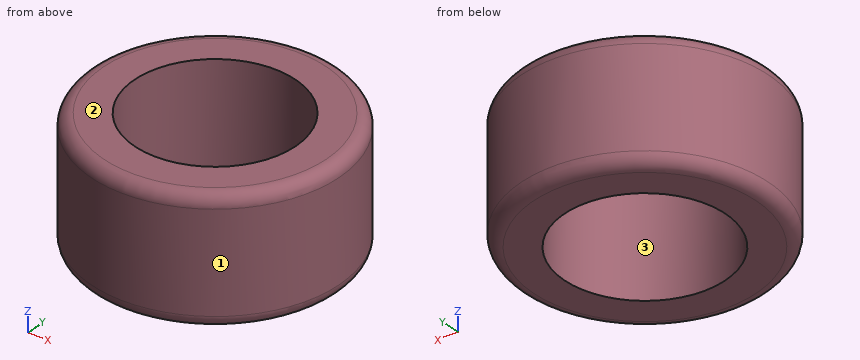
```python
from build123d import *

# Parameters (mm, degrees)
F0_R     = 10
F0_R_2   = 6.5
F1_DEPTH = 10
F2_R     = 1
F3_R     = 1


with BuildPart() as f1:
    # F0 (on Top) → F1 (new body)
    with BuildSketch(Plane.XY):
        Circle(F0_R)
        Circle(F0_R_2, mode=Mode.SUBTRACT)
    extrude(amount=F1_DEPTH)

    # F2
    f2_edges = [f1.edges().sort_by_distance(p)[0] for p in [
        (-10, 0, 10),
    ]]
    fillet(f2_edges, radius=F2_R)

    # F3
    f3_edges = [f1.edges().sort_by_distance(p)[0] for p in [
        (-10, 0, 0),
    ]]
    fillet(f3_edges, radius=F3_R)


solid = f1.part
```
Can you work these out from the model? Positions are in its coordinate system, mm. Face numbers are marked on the shaded views. Round coordinates to 2 decimals unless told otherwise and drop trailing zeros. Loops run counter-clockwise (first coordinate to the right, second up) from the corner with the lowest first, then second, coordinate; pieces in that order, holes last. Notation, with made-up numbers: M 11,13 L 46,13 A25 ccw 46,39 Z; hole C 19.25,-13.75 d3. An arc over 180 degrees is marked long. Write item = value, one per line. Start each with the question number.
(1) If we mould it in two halves opening along X, with no side actions, what happens to the marked faces 1, 2 and 3? For each: released by +X, released by -X, zero draft, split by the parting line, or undercut.
(2) I'm going to push flat-ended pins straight in: P1, Ø6, axis at y = -7.5, z = 4.5, coming from the -X side; P2, Ø1, axis at x = -3.5, z = 4.5, coming from the +Y side; P3, Ø2, axis at y = 1.5, z = 3.5, coming from the -X side. Where does each tip first touch, or does it pass through?
(3) Suppose I cut it at A-A on y = 0. Write out the boundary of the cut face in (x, z).
(4) Suppose I cut it at C-C on z = 8.5. Write out the boundary of the cut face in (x, y).
(5) I need wall thicknesses on line 1 along Y through (x, z) = (0, 5); line 2 along Y through (x, z) = (3, 4); line 3 along X through (y, z) = (0.25, 9.25). Which ranges of each line are inside material? Lowest first, please.
Answer block:
q1.face_1 = split by the parting line
q1.face_2 = zero draft
q1.face_3 = undercut
q2.P1 = -8.93
q2.P2 = 9.54
q2.P3 = -9.99
q3.outline = M -10,1 A1 ccw -9,0 L -6.5,0 L -6.5,10 L -9,10 A1 ccw -10,9 Z; M 6.5,0 L 9,0 A1 ccw 10,1 L 10,9 A1 ccw 9,10 L 6.5,10 Z
q4.outline = C 0,0 d20; hole C 0,0 d13
q5.line_1 = -10 to -6.5, 6.5 to 10
q5.line_2 = -9.54 to -5.77, 5.77 to 9.54
q5.line_3 = -9.97 to -6.5, 6.5 to 9.97
